from build123d import *

# Parameters (mm, degrees)
SKETCH_1_R      = 2.5
EXTRUDE_1_DEPTH = 100
EXTRUDE_2_DEPTH = 3
EXTRUDE_START   = 100
EXTRUDE_3_DEPTH = 3
SKETCH_5_R      = 0.75
EXTRUDE_4_DEPTH = 20


with BuildPart() as part:
    # 草圖1 → 填料-伸長1 (new body)
    with BuildSketch(Plane.XY):
        Circle(SKETCH_1_R)
    extrude(amount=EXTRUDE_1_DEPTH)

    # 草圖3 → 填料-伸長2 (add)
    with BuildSketch(Plane.XY):
        Polygon((1.082752823, 3.893710269), (-2.830675596, 2.884546585), (-3.913428419, -1.009163684), (-1.082752823, -3.893710269), (2.830675596, -2.884546585), (3.913428419, 1.009163684), align=None)
    extrude(amount=-EXTRUDE_2_DEPTH)

    # 草圖4 → 填料-伸長3 (add)
    with BuildSketch(Plane.XY.offset(EXTRUDE_START)):
        Polygon((-2.830675596, 2.884546585), (-3.913428419, -1.009163684), (-1.082752823, -3.893710269), (2.830675596, -2.884546585), (3.913428419, 1.009163684), (1.082752823, 3.893710269), align=None)
    extrude(amount=EXTRUDE_3_DEPTH)

    # 草圖5 → 填料-伸長4 (add)
    with BuildSketch(Plane.XY):
        Circle(SKETCH_5_R)
    extrude(amount=-EXTRUDE_4_DEPTH)


solid = part.part
Build history of the part. All positions in model axes, mm. A direction names the side the tool comes from. Give positions to 0.01 mm unless a question says otherwise; leave off trailing zeros. Loops run counter-clockwise (first coordinate to the right, second up) from the corner with the lowest first, then second, coordinate; pieces in that order, holes last. Notation, with made-up numbers: (40, 16.25) - (71, 16.25) arc R34 cw to (71, 55.25) - close; hole circle Ø2 at (17.5, 54). An arc over 180 degrees is marked (long way). Write item = value, one per line. Start each with the question number.
1) Band-saw the part on A-A on z = 1.5. Give the cut face in (x, y).
2) Tool access for faces 4 (the flat face through (-2.52, -2.43, 101.48)), 5 (the flat face through (-2, 2, 100)): list every direction of +Z, -Z, +X, -X, +Y, -Y with a clear straight run to the whole face (end or side of a thin tool).
3) Pull direction Z, two halves, no side cores. Call faces 1 (the cylindrical face through (-0.54, -2.44, 49.3)), 2 (the flat face through (-3.364, 0.965, -1.479)), 3 (the flat face through (0, 0, 103)): +Z half, -Z half, draft (parallel to the pull), parting line (faces both ways), or undercut.
4) Drop flat-ended pins along their axis: pin 1 Ø3 at (y, z) = (-2.5, 13.5) entering from -X; pin 2 Ø2 at (x, z) = (-2, 72) entering from -Y. Give the stop position or say it passes through.
5) Probe probe 1 along Z at (x, y) = (1.5, 2.75); probe 2 along Y at (x, z) = (-0.25, 73); probe 3 along Z at (x, y) = (-1.5, 0.5). List the from-to ranges inside material, lowest first. Write a range as from..to.
Final values:
q1.outline = circle Ø5 at (0, 0)
q2.face_4 = +Z, -Z, -X, -Y
q2.face_5 = none
q3.face_1 = undercut
q3.face_2 = draft
q3.face_3 = +Z half
q4.pin_1 = -2.29
q4.pin_2 = -2.29
q5.probe_1 = -3..0, 100..103
q5.probe_2 = -2.49..2.49
q5.probe_3 = -3..103
